For this review, take the finished solid that the model builds, in its own axes (mm). A direction names the side the tool comes from. Round coordinates to 2 decimals unless told otherwise and drop trailing zeros. Write each loop counter-clockwise with the first axis right and the second up, starting at its lowest first coordinate (ties: lowest second). Pieces come first, ordered by that corner, then holes. Notation, with made-up numbers: M -31.75,75 L -22.75,75 A20 ccw -22.75,96 Z; hole C 88.25,22.5 d6. An arc over 180 degrees is marked long. Use one line per item in the form item = value. Start each with the question number.
Item 1: Add section A-A (y = 37.9). State the section outline as (x, z) points, and give its area (3 significant figures).
Item 2: For faces 1 (the flat face through (11.5, 26.9, -2)), 2 (the flat face through (14, 26, 44.7)), 3 (the cylindrical face through (4.126, 23.267, -3.514)), list the 3-axis set-ups (+Z, -Z, +X, -X, +Y, -Y) from which the entire face can be reached by the end or side of a thin tool; tool diameter is ignored.
Item 3: Add section D-D (x = 18.25). State the section outline as (y, z) points.
Item 4: Draft analysis for pull direction Z (two halves, no side actions). For faces 4 (the flat face through (10, 30, 46.7)), 5 (the cylindrical face through (1.87, 30.89, -3.51)), 6 (the cylindrical face through (11.61, 32.43, -2.25)), 7 (the cylindrical face through (16.466, 27.219, 41.186)), state which applies: released by +Z, released by -Z, zero draft, split by the parting line, or undercut.
Item 5: For line 1 (Z direction, x = 9.5, y = 24.5); line 2 (Z direction, x = 13.5, y = 31); line 3 (X direction, y = 34, z = 33.5), list the stretches that pass through material, from the lowest coordinate up. Write a range as [from, to].
Item 6: For P1, Ø2.5, axis at x = 15.66, y = 35.56, coming from the +Z side; P2, Ø2, axis at x = 10, y = 18.5, coming from the -Z side; P3, Ø1.6, axis at x = 10, y = 21.9, coming from the +Z side; P4, Ø1.2, axis at x = 18.25, y = 6.35, coming from the -Z side, all flat-tipped, find the tip position at first contact; note any pin that passes through.
Item 7: Add section C-C (z = 35.5). State the section outline as (x, y) points, and give its area (3 significant figures).
Item 8: Add section B-B (x = 14). State the section outline as (y, z) points.
from build123d import *

# Parameters (mm, degrees)
F0_W          = 20
F0_H          = 40.2
F1_DEPTH      = 40.2
F2_R          = 1
F3_DEPTH      = 40.201
F4_R          = 7
F5_DEPTH      = 2
F5_DEPTH_BACK = 42.2
F6_R          = 3
F7_DEPTH      = 2.5
F8_R          = 9.5
F8_R_2        = 1
F9_DEPTH      = 2
F12_R         = 5
F13_DEPTH     = 2


with BuildPart() as f1:
    # F0 (on Top) → F1 (new body)
    with BuildSketch(Plane.XY):
        with Locations((10, 20.1)):
            Rectangle(F0_W, F0_H)
    extrude(amount=F1_DEPTH)

    # F2 (on face) → F3 (cut, through all)
    with BuildSketch(Plane.XY.offset(40.2)):
        with Locations((1.75, 33.85)):
            Circle(F2_R)
        with Locations((18.25, 33.85)):
            Circle(F2_R)
        with Locations((1.75, 6.35)):
            Circle(F2_R)
        with Locations((18.25, 6.35)):
            Circle(F2_R)
    extrude(amount=-F3_DEPTH, mode=Mode.SUBTRACT)

    # F4 (on face) → F5 (join, two sides)
    with BuildSketch(Plane.XY.offset(40.2)) as f5_sk:
        with Locations((10, 29.9)):
            Circle(F4_R)
    extrude(amount=F5_DEPTH)
    extrude(f5_sk.sketch, amount=-F5_DEPTH_BACK)

    # F6 (on face) → F7 (join)
    with BuildSketch(Plane.XY.offset(42.2)):
        with Locations((10, 29.9)):
            Circle(F6_R)
    extrude(amount=F7_DEPTH)

    # F8 (on face) → F9 (join)
    with BuildSketch(Plane.XY.offset(44.7)):
        with Locations((10, 29.9)):
            Circle(F8_R)
        with Locations((4.343146, 24.243146)):
            Circle(F8_R_2, mode=Mode.SUBTRACT)
        with Locations((10, 21.9)):
            Circle(F8_R_2, mode=Mode.SUBTRACT)
        with Locations((15.656854, 24.243146)):
            Circle(F8_R_2, mode=Mode.SUBTRACT)
        with Locations((2, 29.9)):
            Circle(F8_R_2, mode=Mode.SUBTRACT)
        with Locations((4.343146, 35.556854)):
            Circle(F8_R_2, mode=Mode.SUBTRACT)
        with Locations((18, 29.9)):
            Circle(F8_R_2, mode=Mode.SUBTRACT)
        with Locations((10, 37.9)):
            Circle(F8_R_2, mode=Mode.SUBTRACT)
        with Locations((15.656854, 35.556854)):
            Circle(F8_R_2, mode=Mode.SUBTRACT)
    extrude(amount=-F9_DEPTH)

    # F11: F1 across plane


with BuildPart() as f1_1:
    add(f1.part)
    add(f1.part.mirror(Plane.XY.offset(20.1)))

    # F12 (on face) → F13 (join)
    with BuildSketch(Plane.XY.offset(44.7)):
        with Locations((10, 29.9)):
            Circle(F12_R)
    extrude(amount=F13_DEPTH)


solid = f1_1.part
Calculated:
q1.outline = M 0,0 L 20,0 L 20,40.2 L 0,40.2 Z; M 4.88,-4.5 L 9,-4.5 L 9,-2.5 L 4.88,-2.5 Z; M 4.88,42.7 L 9,42.7 L 9,44.7 L 4.88,44.7 Z; M 11,-4.5 L 15.12,-4.5 L 15.12,-2.5 L 11,-2.5 Z; M 11,42.7 L 15.12,42.7 L 15.12,44.7 L 11,44.7 Z
q1.area = 837 mm^2
q2.face_1 = none
q2.face_2 = +Z
q2.face_3 = -Z
q3.outline = M 0,0 L 5.35,0 L 5.35,40.2 L 0,40.2 Z; M 7.35,0 L 32.85,0 L 32.85,40.2 L 7.35,40.2 Z; M 25.19,-4.5 L 28.93,-4.5 L 28.93,-2.5 L 25.19,-2.5 Z; M 25.19,42.7 L 28.93,42.7 L 28.93,44.7 L 25.19,44.7 Z; M 30.87,-4.5 L 34.61,-4.5 L 34.61,-2.5 L 30.87,-2.5 Z; M 30.87,42.7 L 34.61,42.7 L 34.61,44.7 L 30.87,44.7 Z; M 34.85,0 L 40.2,0 L 40.2,40.2 L 34.85,40.2 Z
q4.face_4 = released by +Z
q4.face_5 = zero draft
q4.face_6 = undercut
q4.face_7 = undercut
q5.line_1 = [-4.5, -2.5], [-2, 42.2], [42.7, 44.7]
q5.line_2 = [-4.5, -2.5], [-2, 42.2], [42.7, 46.7]
q5.line_3 = [0, 0.76], [2.74, 17.26], [19.24, 20]
q6.P1 = 44.7
q6.P2 = 0
q6.P3 = 40.2
q6.P4 = through
q7.outline = M 0,0 L 20,0 L 20,40.2 L 0,40.2 Z; hole C 1.75,6.35 d2; hole C 1.75,33.85 d2; hole C 18.25,6.35 d2; hole C 18.25,33.85 d2
q7.area = 791 mm^2
q8.outline = M 0,0 L 24.16,0 L 24.16,-2 L 35.64,-2 L 35.64,0 L 40.2,0 L 40.2,40.2 L 35.64,40.2 L 35.64,42.2 L 24.16,42.2 L 24.16,40.2 L 0,40.2 Z; M 21.28,-4.5 L 38.52,-4.5 L 38.52,-2.5 L 21.28,-2.5 Z; M 21.28,42.7 L 38.52,42.7 L 38.52,44.7 L 32.9,44.7 L 32.9,46.7 L 26.9,46.7 L 26.9,44.7 L 21.28,44.7 Z
